Check sheet for the drawn part. Datum: minimum x, y, z corner. Units: mm. A direction names the side the tool comes from. Coordinates: 2 decimals unless noted, no trailing zeros. Loops run counter-clockwise (first coordinate to the right, second up) from the corner with the lowest first, then second, coordinate; pieces in that order, holes last. Notation, with made-up numbers: M 47,28 L 65,28 A24 cw 65,47 Z; hole C -16.75,11.25 d11. An arc over 180 degrees is marked long. Use CSV: the item, a comma, the result in double quotes. Start each with the question number.
(1) Section check B-B on z = 17. Record the cut outline in (x, y).
(2) Scan lines: line 1 (X direction, y = 25, z = 15.75); line 2 (Y direction, x = 12.5, z = 12.75); line 3 (Z direction, x = 35.5, y = 2). Record each from-to range of solid material in increasing order.
(3) Section check C-C on z = 27. Record the cut outline in (x, y), and give its area (3 significant figures).
(4) Set-up check for the marked faces 4, 5 and 6: record each of +Z, -Z, +X, -X, +Y, -Y from which the full face is reachable in a straight line by a thin tool's end or side.
(5) Go/stop test with flat-tipped pins: pin 1 Ø4 at (y, z) = (42.5, 5.5) entering from +X; pin 2 Ø19 at (x, y) = (57.5, 25) entering from +Z; pin 3 Ø6 at (y, z) = (20, 25.5) entering from -X. Record where each tip stops, or that it passes through.
(6) Draft check along X on the marked faces 1, 2 and 3. Enter one of: pulls with the +X half, pulls with the -X half, needs draft (parallel to the pull), parting line crosses it, or undercut.
(7) Section check A-A on x = 57.5. Record the cut outline in (y, z).
(8) Section check D-D on x = 16.5. Record the cut outline in (y, z), and give its area (3 significant figures).
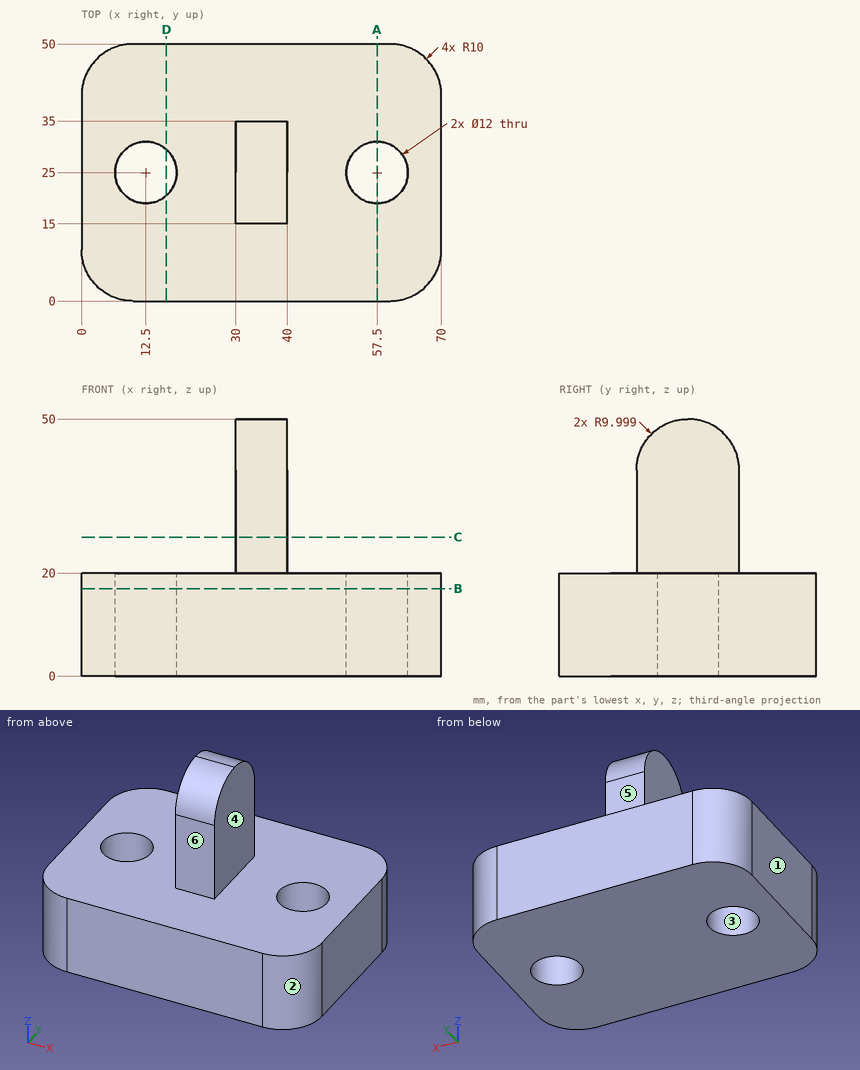
Outcome:
1,outline,"M 0,10 A10 ccw 10,0 L 60,0 A10 ccw 70,10 L 70,40 A10 ccw 60,50 L 10,50 A10 ccw 0,40 Z; hole C 12.5,25 d12; hole C 57.5,25 d12"
2,line 1,"x = 0 to 6.5, 18.5 to 51.5, 63.5 to 70"
2,line 2,"y = 0 to 19, 31 to 50"
2,line 3,"z = 0 to 20"
3,outline,"M 30,15 L 40,15 L 40,35 L 30,35 Z"
3,area,"200 mm²"
4,face 4,"+Z, +X, +Y, -Y"
4,face 5,"+Z, +X, -X, +Y"
4,face 6,"+Z, +X, -X, -Y"
5,pin 1,"stops at x = 69.99"
5,pin 2,"stops at z = 20"
5,pin 3,"stops at x = 30"
6,face 1,"pulls with the -X half"
6,face 2,"pulls with the +X half"
6,face 3,"undercut"
7,outline,"M 0,0 L 19,0 L 19,20 L 0,20 Z; M 31,0 L 50,0 L 50,20 L 31,20 Z"
8,outline,"M 0,0 L 20.53,0 L 20.53,20 L 0,20 Z; M 29.47,0 L 50,0 L 50,20 L 29.47,20 Z"
8,area,"821 mm²"
